Work out the finished part from the listing and answer in its coordinate system (mm). A direction names the side the tool comes from. Coordinates: 2 decimals unless noted, no trailing zeros. Loops run counter-clockwise (first coordinate to the right, second up) from the corner with the lowest first, then second, coordinate; pieces in that order, holes last. Notation, with made-up numbers: (19, 63) - (37, 63) arc R19 cw to (37, 86) - close; hole circle Ø8 at (55.25, 16). An arc over 180 degrees is marked (long way). Write each question's results on one line, items separated by ' | '. Start each with the question number.
1. A cutting plane is placed at A-A on z = 182. Determine the outline of the cut face in (x, y), then the cut area to 3 significant figures.
2. Find the intervals of material crossed by line 1 along Y through (x, z) = (-8.35, 70); line 2 along Y through (x, z) = (5.25, 27.5), in increasing order. Write a range as [from, to].
3. Which of the six approach directions +Z, -Z, +X, -X, +Y, -Y give full straight-line access (tool end or side, diameter ignored) to faces 1 (the flat face through (-10, 0, 227)), 2 (the flat face through (0, 8, 227))?
4. Determine the mould class of faces 3 (the flat face through (0, 10, 227)), 4 (the flat face through (-9, 0, 460)), 5 (the flat face through (0, -10, 227)), 6 (the flat face through (-8, 0, 227)) for opening direction Y: released by +Y, released by -Y, zero draft, split by the parting line, or undercut.
from build123d import *

# Parameters (mm, degrees)
SKETCH_1_W          = 20
SKETCH_1_H          = 20
SKETCH_1_W_2        = 16
SKETCH_1_H_2        = 16
EXTRUDE_1_DEPTH     = 460
SKETCH_2_R          = 2
CUT_EXTRUDE_1_DEPTH = 461.543157587
SKETCH_3_R          = 2
CUT_EXTRUDE_2_DEPTH = 461.543157587


with BuildPart() as part:
    # 草图1 → 凸台-拉伸1 (new body)
    with BuildSketch(Plane.XY):
        Rectangle(SKETCH_1_W, SKETCH_1_H)
        Rectangle(SKETCH_1_W_2, SKETCH_1_H_2, mode=Mode.SUBTRACT)
    extrude(amount=EXTRUDE_1_DEPTH)

    # 草图2 → 切除-拉伸1 (cut, through all)
    with BuildSketch(Plane(origin=(10, 0, 0), x_dir=(0, 0, -1), z_dir=(1, 0, 0))):
        with Locations((-450, 0)):
            Circle(SKETCH_2_R)
        with Locations((-70, 0)):
            Circle(SKETCH_2_R)
        with Locations((-110, 0)):
            Circle(SKETCH_2_R)
        with Locations((-150, 0)):
            Circle(SKETCH_2_R)
        with Locations((-37.153023279, -18.374821325)):
            Circle(SKETCH_2_R)
        with Locations((-17.227343837, -16.652236413)):
            Circle(SKETCH_2_R)
        with Locations((-430.074320558, 1.722584912)):
            Circle(SKETCH_2_R)
    extrude(amount=-CUT_EXTRUDE_1_DEPTH, mode=Mode.SUBTRACT)

    # 草图3 → 切除-拉伸2 (cut, through all)
    with BuildSketch(Plane(origin=(0, 10, 0), x_dir=(1, 0, 0), z_dir=(0, 1, 0))):
        with Locations(Location((0, -260, 0), (0, 0, 270))):
            Circle(SKETCH_3_R)
        with Locations(Location((0, -300, 0), (0, 0, 270))):
            Circle(SKETCH_3_R)
    extrude(amount=-CUT_EXTRUDE_2_DEPTH, mode=Mode.SUBTRACT)


solid = part.part
Values:
1) outline: (-10, -10) - (10, -10) - (10, 10) - (-10, 10) - close; hole (-8, -8) - (8, -8) - (8, 8) - (-8, 8) - close | area: 144 mm^2
2) line 1: [-10, -2], [2, 10] | line 2: [-10, -8], [8, 10]
3) face 1: +Z, -Z, -X, +Y, -Y | face 2: +Z, -Z
4) face 3: released by +Y | face 4: zero draft | face 5: released by -Y | face 6: undercut
